Read the model definition and answer for the solid it produces. Units are mm, in the model's axes. A direction names the side the tool comes from. Give positions to 0.01 mm unless a question says otherwise; leave off trailing zeros. Order: outer loops, then holes, each group sorted by start corner. A loop starts at its lowest first (then second) coordinate and runs counter-clockwise, first axis right, second up.
Item 1: A cutting plane is placed at D-D (y = 6.5). Write down the section's boundary in (x, z).
Item 2: Which of the six approach directions +Z, -Z, +X, -X, +Y, -Y give full straight-line access (tool end or side, diameter ignored) to faces 5 (the face through (-8, -82.25, -10)), 6 (the face through (2.46, -88.86, 6.92)), 7 (the face through (2, -1, 15)), 8 (the face through (-2.7, -1.2, -5)), 9 (the face through (-9, -1, -7))?
Item 3: A cutting plane is placed at A-A (x = -10.75). Write down the section's boundary in (y, z), plus the area to 3 significant figures.
Item 4: Given pin 1 Ø10 at (x, z) = (-15.5, 3.5) entering from -Y; pin 2 Ø1 at (x, y) = (-13, -60.5) entering from +Z; pin 3 Ø13.5 at (x, y) = (-11, 14.5) entering from +Z; pin 4 Ø8 at (x, z) = (-11, 29) entering from +Y, each flat-ended and moving along its own axis, determine where each tip first touches the part or whether it passes through.
Item 5: A cutting plane is placed at C-C (y = -85). Write down the section's boundary in (x, z).
Item 6: A cutting plane is placed at B-B (z = 2). Write down the section's boundary in (x, y).
Item 7: The mould has two halves that part along Y. Classify faces 1 (the face through (-19.46, 89.83, 44.65)), 2 (the face through (2.46, 89.83, 44.65)), 3 (the face through (2.46, 89, 7.56)), 4 (the face through (0, 1.3, 14.6)): +Y half, -Y half, draft (parallel to the pull), parting line (faces both ways), or undercut.
Item 8: Find the intervals of material crossed by line 1 along Z through (x, y) = (-16.25, -38); line 2 along Z through (x, y) = (-11.5, 28.5); line 3 along Y through (x, z) = (-7.75, -5.5), in increasing order.
from build123d import *

# Parameters (mm, degrees)
SALIENTE_EXTRUIR1_DEPTH = 5
CROQUIS3_W              = 10
CROQUIS3_H              = 164.5
SALIENTE_EXTRUIR2_DEPTH = 10
VACIADO1_START          = -74.25
VACIADO1_OUTLINE_W      = 11
VACIADO1_OUTLINE_H      = 2
VACIADO1_DEPTH          = 148.5


# Read off the part's stored shape, not the designer's step: Vaciado1
with BuildPart() as part:
    # Croquis1 → Saliente-Extruir1 (new body)
    with BuildSketch(Plane(origin=(0, 0, 0), x_dir=(0, 0, -1), z_dir=(1, 0, 0))):
        with BuildLine():
            Line((-29.506547344, 95.56963472), (15, 82.25))
            Line((15, 82.25), (15, -82.25))
            Line((15, -82.25), (-29.472062031, -95.659500692))
            ThreePointArc((-29.472062031, -95.659500692), (-44.574231242, -90.213203382), (-35, -77.326319918))
            Line((-35, -77.326319918), (-15, -67.539809421))
            Line((-15, -67.539809421), (-15, 67.43308889))
            Line((-15, 67.43308889), (-35, 77.213680082))
            ThreePointArc((-35, 77.213680082), (-44.580176052, 90.080773873), (-29.506547344, 95.56963472))
        make_face()
    extrude(amount=SALIENTE_EXTRUIR1_DEPTH)


with BuildPart() as body_2:
    # Simetría3: mirrored copy
    add(part.part.mirror(Plane(origin=(-8.5, 0, 0), x_dir=(0, 0, 1), z_dir=(1, 0, 0))))


with BuildPart() as part_1:
    add(part.part)

    add(body_2.part)  # Saliente-Extruir2 merges body 2
    # Croquis3 → Saliente-Extruir2 (add, symmetric)
    with BuildSketch(Plane(origin=(-8.5, 0, 0), x_dir=(0, 0, -1), z_dir=(1, 0, 0))):
        with Locations((10, 0)):
            Rectangle(CROQUIS3_W, CROQUIS3_H)
    extrude(amount=SALIENTE_EXTRUIR2_DEPTH, both=True)

    # Vaciado1 outline → Vaciado1 (cut)
    with BuildSketch(Plane(origin=(0, 0, 0), x_dir=(1, 0, 0), z_dir=(0, 1, 0)).offset(VACIADO1_START)):
        with Locations((-8.5, 6)):
            Rectangle(VACIADO1_OUTLINE_W, VACIADO1_OUTLINE_H)
    extrude(amount=VACIADO1_DEPTH, mode=Mode.SUBTRACT)


solid = part_1.part
Response values:
1. outline: (-22, -15) - (5, -15) - (5, 15) - (0, 15) - (0, -5) - (-3, -5) - (-3, -7) - (-14, -7) - (-14, -5) - (-17, -5) - (-17, 15) - (-22, 15) - close
2. face 5: +Z, -Z, -Y
2. face 6: -Z, +X, -X, -Y
2. face 7: +Z, +X, -X
2. face 8: +Z, +Y, -Y
2. face 9: +Z
3. outline: (-82.25, -15) - (82.25, -15) - (82.25, -5) - (74.25, -5) - (74.25, -7) - (-74.25, -7) - (-74.25, -5) - (-82.25, -5) - close
3. area: 1,350 mm2
4. pin 1: stops at y = -89.27
4. pin 2: stops at z = -7
4. pin 3: stops at z = 15
4. pin 4: passes through
5. outline: (-22, -5.88) - (-17, -5.88) - (-17, 44.73) - (-22, 44.73) - close; (0, -5.88) - (5, -5.88) - (5, 44.73) - (0, 44.73) - close
6. outline: (-22, -87.38) - (-17, -87.38) - (-17, 87.34) - (-22, 87.34) - close; (0, -87.38) - (5, -87.38) - (5, 87.34) - (0, 87.34) - close
7. face 1: undercut
7. face 2: undercut
7. face 3: +Y half
7. face 4: draft
8. line 1: z = -15 to -5
8. line 2: z = -15 to -7
8. line 3: y = -82.25 to -74.25, 74.25 to 82.25
